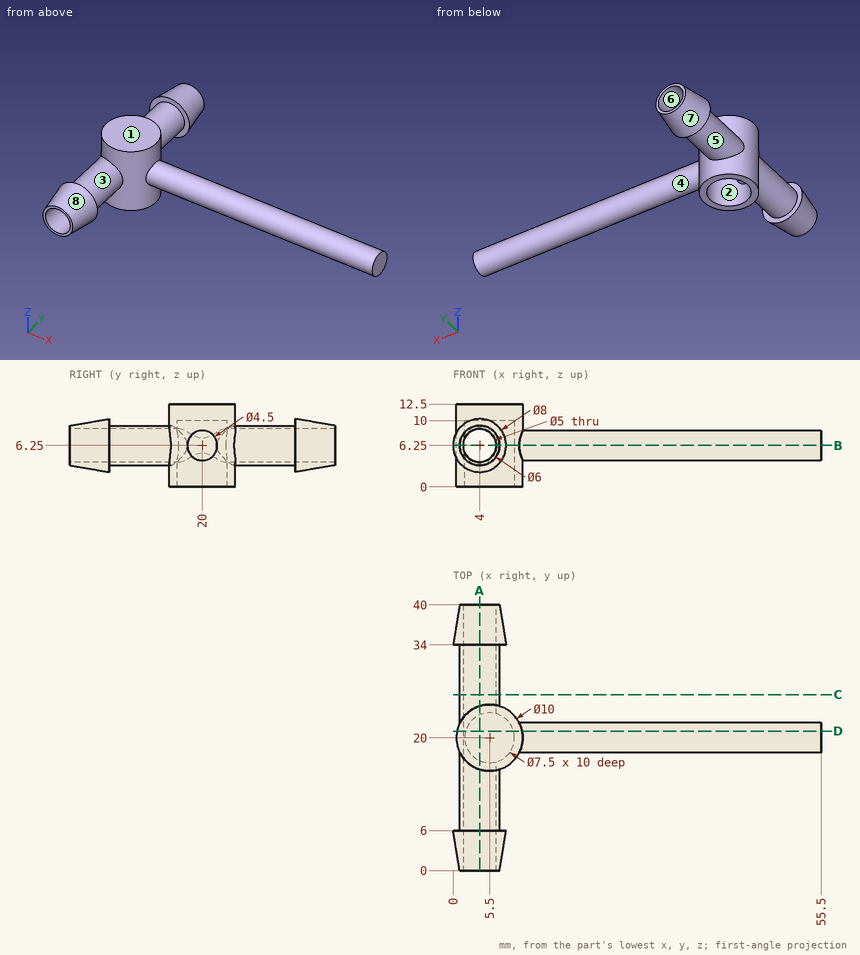
Study the drawing (mm; zero at the part's minimum x, y, z) and answer. A direction names the side the tool comes from. Give positions to 0.01 mm unless a question says otherwise; leave off trailing zeros. Write each loop counter-clockwise with the first axis right and the second up, starting at its lowest first coordinate (ties: lowest second). Pieces come first, ordered by that corner, then holes. Notation, with made-up numbers: (-12.5, 74) -> (-4.5, 74) arc R20 cw to (-4.5, 79) -> close; hole circle Ø2 at (-10, 39). An arc over 180 degrees is marked (long way). Write item = value, one per line.
Q1. Section D-D on y = 21 is taken. Determine the outline of the cut face in (x, z), and give its area (3 significant figures).
Computed values:
outline = (0.6, 0) -> (1.89, 0) -> (1.89, 4.92) arc R2.5 cw to (1.89, 7.58) -> (1.89, 10) -> (9.11, 10) -> (9.11, 0) -> (10.4, 0) -> (10.4, 4.23) -> (55.5, 4.23) -> (55.5, 8.27) -> (10.4, 8.27) -> (10.4, 12.5) -> (0.6, 12.5) -> close
area = 231 mm^2
Q2. For a pull along Y with two mould halves and no side action, classify the marked faces 5, 6, 7 and 8 as pulls with the +Y half, pulls with the -Y half, needs draft (parallel to the pull), parting line crosses it, or undercut.
Computed values:
face_5 = undercut
face_6 = needs draft
face_7 = pulls with the +Y half
face_8 = pulls with the -Y half
Q3. Section A-A on x = 4 is taken. State how many separate pieces and enclosed holes the cut face has, and give its area (3 significant figures).
Computed values:
separate_pieces = 3
enclosed_holes = 0
area = 79.6 mm^2
Q4. Section B-B on z = 6.25 is taken. Determine the outline of the cut face in (x, y).
Computed values:
outline = (0, 6) -> (1, 0) -> (1.5, 0) -> (1.5, 40) -> (1, 40) -> (0, 34) -> (1, 34) -> (1, 22.18) arc R5 ccw to (1, 17.82) -> (1, 6) -> close; (6.5, 0) -> (7, 0) -> (8, 6) -> (7, 6) -> (7, 15.23) arc R5 ccw to (9.97, 17.75) -> (55.5, 17.75) -> (55.5, 22.25) -> (9.97, 22.25) arc R5 ccw to (7, 24.77) -> (7, 34) -> (8, 34) -> (7, 40) -> (6.5, 40) -> (6.5, 23.61) arc R3.75 cw to (6.5, 16.39) -> close
Q5. Consider line 1 along Y through (x, z) = (5.5, 3.75); line 2 along Z through (x, y) = (4, 15); line 3 along Y through (x, z) = (48.5, 6.5). Determine where each line is inside the solid, lowest interval first.
Computed values:
line_1 = 0 to 16.25, 23.75 to 40
line_2 = 3.25 to 3.75, 8.75 to 9.25
line_3 = 17.76 to 22.24
Q6. Flat-ended cylindrical pins translate along their axes: pin 1 Ø12 at (x, y) = (46, 32) entering from -Z; pin 2 Ø2 at (x, y) = (7, 19) entering from -Z; pin 3 Ø5 at (x, y) = (6, 5) entering from -Z; pin 4 Ø3 at (x, z) = (30, 6) entering from -Y. Find the tip coordinate at first contact, or state that the pin passes through.
Computed values:
pin_1 = through
pin_2 = 10
pin_3 = 2.25
pin_4 = 17.75
Q7. Section C-C on y = 26.5 is taken. Determine the outline of the cut face in (x, z).
Computed values:
outline = circle Ø6 at (4, 6.25); hole circle Ø5 at (4, 6.25)
Q8. A tool of negligible diameter and unlimited length cuts with its end or side. For the marked faces 1, 2, 3 and 4, from which of +Z, -Z, +X, -X, +Y, -Y can it reach the whole face along a straight path? Write none if from no direction.
Computed values:
face_1 = +Z, +X, -X, +Y, -Y
face_2 = -Z
face_3 = none
face_4 = +X
